Autodesk Inventor part; units mm, degrees
ref_plane "YZ Plane" through (0, 0, 0) normal (1, 0, 0) x (0, 1, 0)
ref_plane "XZ Plane" through (0, 0, 0) normal (0, 1, 0) x (-1, 0, 0)
ref_plane "XY Plane" through (0, 0, 0) normal (0, 0, 1) x (1, 0, 0)
sketch "Sketch2" plane through (0, 0, 0) normal (0, 1, 0) x (-1, 0, 0)
  line L0 (0, 0) -> (-36, 0)
  line L1 (-36, 0) -> (-36, -100)
  line L2 (-36, -100) -> (0, -100)
  line L3 (0, -100) -> (0, 0)
  line L4 (-36, 0) -> (-36, -20)
  line L5 (-36, -20) -> (0, -20)
  line L6 (-36, -100) -> (-36, -80)
  line L7 (-36, -80) -> (-36, -61.7109)
  line L8 (0, -61.7109) -> (0, -80)
  line L9 (-36, -80) -> (-36, -70)
  line L10 (-36, -70) -> (0, -70)
  line L11 (0, -80) -> (-36, -80)
  line L12 (0, -70) -> (0, -80)
  line L13 (0, -70) -> (-5, -70)
  line L14 (-5, -70) -> (-5, -80)
  line L15 (-36, -20) -> (-36, -30)
  line L16 (-36, -30) -> (0, -30)
  line L17 (0, -20) -> (-5, -20)
  line L18 (-5, -20) -> (-5, -30)
  line L19 (-36, -80) -> (-31, -80)
  line L20 (-31, -80) -> (-31, -70)
  line L21 (-31, -30) -> (-31, -20)
  line L22 (-18, 0) -> (-18, -15)
  line L23 (-18, -15) -> (-18, -43.5)
  circle A0 centre (-18, -43.5) radius 5.05
  line L24 (-18, -43.5) -> (-18, -82)
  circle A1 centre (-18, -82) radius 5.05
  circle A2 centre (-18, -15) radius 5
  dimension "d0" = 36
  dimension "d1" = 100
  dimension "d2" = 20
  dimension "d3" = 20
  dimension "d4" = 10
  dimension "d5" = 5
  dimension "d6" = 10
  dimension "d7" = 5
  dimension "d8" = 5
  dimension "d9" = 15
  dimension "d11" = 28.5
  dimension "d12" = 10.1
  dimension "d13" = 38.5
  dimension "d14" = 10.1
extrude "Extrusion1" add sketch "Sketch2" along normal blind 5 contours L3 L5 A2 L22 L0 | L22 A2 L5 L1 L0 | L3 L10 L24 A0 L23 L16 | L18 L16 L23 L5 | L23 L16 L21 L5 | L16 L23 A0 L24 L10 L1 | L3 L2 L1 L11 A1 | L14 L11 A1 L24 L10 | L24 A1 L11 L20 L10
equation "\"BendRadius\" = Thickness"
equation "\"BendReliefWidth\" = Thickness"
equation "\"BendReliefDepth\" = 0.5 * Thickness"
equation "\"CornerReliefSize\" = 4 * Thickness"
equation "\"MinimumRemnant\" = 2 * Thickness"
equation "\"TransitionRadius\" = BendRadius"
equation "\"JacobiRadiusSize\" = BendRadius"
equation "\"GapSize\" = Thickness"
Source: CAD feature listing. Evaluate the final solid. Frame: model axes, mm. A direction names the side the tool comes from. Give positions to 0.01 mm unless a question says otherwise; leave off trailing zeros. Loops run counter-clockwise (first coordinate to the right, second up) from the corner with the lowest first, then second, coordinate; pieces in that order, holes last. Notation, with made-up numbers: (-17, 29.25) -> (14, 29.25) arc R17 ccw to (14, 52.25) -> close; hole circle Ø9 at (-11.75, -32). An arc over 180 degrees is marked (long way). Use a Markdown table: item, result. Add a question column.
1) Line query: line 1 along Z through (x, y) = (18, 3.45); line 2 along Z through (x, y) = (34, 4.7); line 3 along X through (y, z) = (1.7, -15). Output: solid intervals per line, ascending. Write a range as [from, to].
2) First-contact query: pin 1 (1.5 mm diameter, centred on x = 30, z = -87.5, fed in from -Y); pin 2 (3 mm diameter, centred on y = 4, z = -24, fed in from -X). Flat tips, straight axial feed; report the tip coordinate or a pass-through.
3) Section query D-D, the plane z = -15. Return the cut outline in (x, y).
4) Section query B-B, the plane x = 18. Return the cut outline in (y, z).
5) Section query A-A, the plane z = -82. Return the cut outline in (x, y).
6) Section query C-C, the plane y = 1.4. Return the cut outline in (x, z), then the cut area to 3 significant figures.
7) Reachability of faces 1 (the face through (0, 2, -10)), 2 (the face through (5, 2, -75)), 3 (the face through (34, 2, -20)) from +Z, -Z, +X, -X, +Y, -Y: full face, straight path, thin tool, end or side. Return the list, or none.
Numbers:
| question | item | result |
|---|---|---|
| 1 | line 1 | z = [-100, -87.05], [-76.95, -48.55], [-38.45, -20], [-10, 0] |
| 1 | line 2 | z = [-100, -80], [-70, -30], [-20, 0] |
| 1 | line 3 | x = [0, 13], [23, 36] |
| 2 | pin 1 | stops at y = 0 |
| 2 | pin 2 | stops at x = 5 |
| 3 | outline | (0, 0) -> (13, 0) -> (13, 5) -> (0, 5) -> close; (23, 0) -> (36, 0) -> (36, 5) -> (23, 5) -> close |
| 4 | outline | (0, -100) -> (5, -100) -> (5, -87.05) -> (0, -87.05) -> close; (0, -76.95) -> (5, -76.95) -> (5, -48.55) -> (0, -48.55) -> close; (0, -38.45) -> (5, -38.45) -> (5, -20) -> (0, -20) -> close; (0, -10) -> (5, -10) -> (5, 0) -> (0, 0) -> close |
| 5 | outline | (0, 0) -> (12.95, 0) -> (12.95, 5) -> (0, 5) -> close; (23.05, 0) -> (36, 0) -> (36, 5) -> (23.05, 5) -> close |
| 6 | outline | (0, -100) -> (36, -100) -> (36, -80) -> (31, -80) -> (31, -70) -> (36, -70) -> (36, -30) -> (31, -30) -> (31, -20) -> (36, -20) -> (36, 0) -> (0, 0) -> (0, -20) -> (5, -20) -> (5, -30) -> (0, -30) -> (0, -70) -> (5, -70) -> (5, -80) -> (0, -80) -> close; hole circle Ø10.1 at (18, -82); hole circle Ø10.1 at (18, -43.5); hole circle Ø10 at (18, -15) |
| 6 | area | 3,160 mm2 |
| 7 | face 1 | +Z, -Z, -X, +Y, -Y |
| 7 | face 2 | -X, +Y, -Y |
| 7 | face 3 | +X, +Y, -Y |
